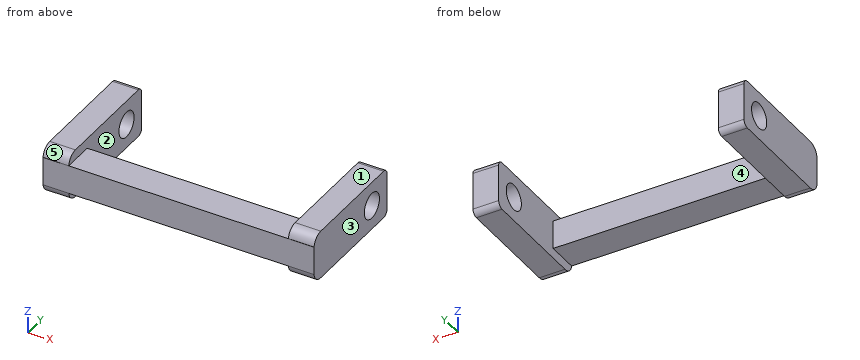
```python
from build123d import *

# Parameters (mm, degrees)
F0_W     = 43
F0_H     = 5.5
F1_DEPTH = 5
F3_DEPTH = 4.5
F5_DEPTH = 4.5
F6_R     = 2.25
F7_DEPTH = 47.501


with BuildPart() as f1:
    # F0 (on Top) → F1 (new body)
    with BuildSketch(Plane.XY):
        with Locations((21.5, 2.75)):
            Rectangle(F0_W, F0_H)
    extrude(amount=F1_DEPTH)

    # F2 (on Right) → F3 (join)
    with BuildSketch(Plane.YZ):
        with BuildLine():
            ThreePointArc((0, 0.25), (0.585786, -1.164214), (2, -1.75))
            Line((2, -1.75), (20.7, -1.75))
            ThreePointArc((20.7, -1.75), (21.407107, -1.457107), (21.7, -0.75))
            Line((21.7, -0.75), (21.7, 5.75))
            ThreePointArc((21.7, 5.75), (21.407107, 6.457107), (20.7, 6.75))
            Line((20.7, 6.75), (2, 6.75))
            ThreePointArc((2, 6.75), (0.585786, 6.164214), (0, 4.75))
            Line((0, 4.75), (0, 0.25))
        make_face()
    extrude(amount=F3_DEPTH)

    # F4 (on face) → F5 (join)
    with BuildSketch(Plane.YZ.offset(43)):
        with BuildLine():
            Line((0.015687, 5), (0, 5))
            Line((0, 5), (0, 0))
            Line((0, 0), (0.015687, 0))
            ThreePointArc((0.015687, 0), (0.677124, -1.25), (2, -1.75))
            Line((2, -1.75), (20.7, -1.75))
            ThreePointArc((20.7, -1.75), (21.407107, -1.457107), (21.7, -0.75))
            Line((21.7, -0.75), (21.7, 5.75))
            ThreePointArc((21.7, 5.75), (21.407107, 6.457107), (20.7, 6.75))
            Line((20.7, 6.75), (2, 6.75))
            ThreePointArc((2, 6.75), (0.677124, 6.25), (0.015687, 5))
        make_face()
    extrude(amount=F5_DEPTH)

    # F6 (on face) → F7 (cut, through all)
    with BuildSketch(Plane(origin=(0, 0, 0), x_dir=(0, -1, 0), z_dir=(-1, 0, 0))):
        with Locations((-17.2, 2.5)):
            Circle(F6_R)
    extrude(amount=-F7_DEPTH, mode=Mode.SUBTRACT)


solid = f1.part
```
Model file for the job. Use its own axes, mm. Face numbers are marked on the shaded views. A direction names the side the tool comes from. Coordinates: 2 decimals unless noted, no trailing zeros. Loops run counter-clockwise (first coordinate to the right, second up) from the corner with the lowest first, then second, coordinate; pieces in that order, holes last. Notation, with made-up numbers: (8.5, 46) - (34.5, 46) arc R20 cw to (34.5, 56) - close; hole circle Ø3 at (4, 37). An arc over 180 degrees is marked (long way). Answer as a JSON object with one key per item and string values. Group by question number.
(1) Flat gauge pins, fed straight in: pin 1 (8 mm diameter, centred on x = 37, y = 5, fed in from +Z); pin 2 (1.5 mm diameter, centred on x = 21, z = 1.5, fed in from +Y); pin 3 (6 mm diameter, centred on x = 12.5, y = 3, fed in from -Z). Where does each tip first touch, or does it go through?
(2) Cut at D-D (z = 6.25). Give the cut face in (x, y).
(3) Tool access for the marked faces 4 and 5: list every direction of +Z, -Z, +X, -X, +Y, -Y with a clear straight run to the whole face (end or side of a thin tool).
(4) Cut at B-B (y = 17.2). Give the cut face in (x, z).
(5) Probe line 1 along X through (y, z) = (6.75, 1.5); line 2 along Z through (x, y) = (3.1, 17.2); line 3 along Y through (x, z) = (21.5, 2.25). List the from-to ranges inside material, lowest first.
(6) Two-plate mould, pull along X, no slides. Class the marked faces 1, 2 and 3: released by +X, released by -X, zero draft, split by the parting line, or undercut.
(7) Cut at C-C (z = 2.5). Give the cut face in (x, y), then the cut area to 3 significant figures.
Geometry says:
{
 "1": {"pin 1": "stops at z = 5", "pin 2": "stops at y = 5.5", "pin 3": "stops at z = 0"},
 "2": {"outline": "(0, 0.68) - (4.5, 0.68) - (4.5, 21.57) - (0, 21.57) - close; (43, 0.68) - (47.5, 0.68) - (47.5, 21.57) - (43, 21.57) - close"},
 "3": {"face 4": "+Z, -Z, +Y", "face 5": "+Z, +X, -X, -Y"},
 "4": {"outline": "(0, -1.75) - (4.5, -1.75) - (4.5, 0.25) - (0, 0.25) - close; (0, 4.75) - (4.5, 4.75) - (4.5, 6.75) - (0, 6.75) - close; (43, -1.75) - (47.5, -1.75) - (47.5, 0.25) - (43, 0.25) - close; (43, 4.75) - (47.5, 4.75) - (47.5, 6.75) - (43, 6.75) - close"},
 "5": {"line 1": "x = 0 to 4.5, 43 to 47.5", "line 2": "z = -1.75 to 0.25, 4.75 to 6.75", "line 3": "y = 0 to 5.5"},
 "6": {"face 1": "zero draft", "face 2": "undercut", "face 3": "released by +X"},
 "7": {"outline": "(0, 0) - (47.5, 0) - (47.5, 14.95) - (43, 14.95) - (43, 5.5) - (4.5, 5.5) - (4.5, 14.95) - (0, 14.95) - close; (0, 19.45) - (4.5, 19.45) - (4.5, 21.7) - (0, 21.7) - close; (43, 19.45) - (47.5, 19.45) - (47.5, 21.7) - (43, 21.7) - close", "area": "367 mm^2"}
}
